```python
from build123d import *

# Parameters (mm, degrees)
SKETCH1_R                     = 39.878
HOUSING_FITTING_EXTRUDE_DEPTH = 17.018
HOUSING_BODY_1_DEPTH          = 19.05
SKETCH3_R                     = 8.509
IMPELLER_BORE_DEPTH           = 17.018
SKETCH4_R                     = 4
SHAFT_BORE_DEPTH              = 70.612
O_RING_CUT_DEPTH              = 1.27
O_RING_CUT_DEPTH_BACK         = 1.27
SKETCH5_R                     = 39.878
SKETCH5_R_2                   = 38.608
SEAL_START                    = 19.05
SKETCH7_R                     = 39.878
SKETCH7_R_2                   = 4
SEAL_SIDE_BODY_EXT_DEPTH      = 19.05
EXT_FILLET_R                  = 5.08
SKETCH10_W                    = 19.05
SKETCH10_H                    = 50.8
DISCHARGE_CUT_DEPTH           = 10.541
SKETCH11_R                    = 19.05
CUT_EXTRUDE1_DEPTH            = 27.94
SKETCH12_R                    = 3.175
CUT_EXTRUDE2_DEPTH            = 19.05
CIRPATTERN1_COUNT             = 8


with BuildPart() as part:
    # Sketch1 → Housing Fitting Extrude (new body)
    with BuildSketch(Plane(origin=(0, 0, 0), x_dir=(0, 0, -1), z_dir=(1, 0, 0))):
        Circle(SKETCH1_R)
    extrude(amount=HOUSING_FITTING_EXTRUDE_DEPTH)

    # Sketch2 → Housing Body 1 (add)
    with BuildSketch(Plane.ZY):
        with BuildLine():
            Line((60.96, 0), (60.96, 60.96))
            Line((60.96, 60.96), (0, 60.96))
            ThreePointArc((0, 60.96), (-43.105229381, 43.105229381), (-60.96, 0))
            Line((-60.96, 0), (-60.96, -54.61))
            Line((-60.96, -54.61), (-60.96, -60.96))
            Line((-60.96, -60.96), (60.96, -60.96))
            Line((60.96, -60.96), (60.96, -54.61))
            Line((60.96, -54.61), (60.96, 0))
        make_face()
    extrude(amount=HOUSING_BODY_1_DEPTH)

    # Sketch3 → Impeller Bore (cut)
    with BuildSketch(Plane(origin=(17.018, 0, 0), x_dir=(0, 0, -1), z_dir=(1, 0, 0))):
        Circle(SKETCH3_R)
    extrude(amount=-IMPELLER_BORE_DEPTH, mode=Mode.SUBTRACT)

    # Sketch4 → Shaft Bore (cut)
    with BuildSketch(Plane(origin=(0, 0, 0), x_dir=(0, 0, -1), z_dir=(1, 0, 0))):
        Circle(SKETCH4_R)
    extrude(amount=-SHAFT_BORE_DEPTH, mode=Mode.SUBTRACT)

    # Sketch5 → O-Ring Cut (cut, two sides: drawn at the far end of the back side and taken through both)
    with BuildSketch(Plane(origin=(8.509, 0, 0), x_dir=(0, 0, -1), z_dir=(1, 0, 0)).offset(-O_RING_CUT_DEPTH_BACK)):
        Circle(SKETCH5_R)
        Circle(SKETCH5_R_2, mode=Mode.SUBTRACT)
    extrude(amount=O_RING_CUT_DEPTH + O_RING_CUT_DEPTH_BACK, mode=Mode.SUBTRACT)

    # Sketch7 → Seal Side Body Ext (add)
    with BuildSketch(Plane.ZY.offset(19.05).offset(SEAL_START)):
        with Locations(Location((0, 0, 0), (0, 0, 180))):
            Circle(SKETCH7_R)
        with Locations(Location((0, 0, 0), (0, 0, 180))):
            Circle(SKETCH7_R_2, mode=Mode.SUBTRACT)
    extrude(amount=-SEAL_SIDE_BODY_EXT_DEPTH)

    # Ext Fillet
    ext_fillet_edges = [part.edges().sort_by_distance(p)[0] for p in [
        (-38.1, 0, 39.878),
        (-19.05, 0, 39.878),
    ]]
    fillet(ext_fillet_edges, radius=EXT_FILLET_R)

    # Sketch10 → Discharge Cut (cut)
    with BuildSketch(Plane.XY.offset(60.96)):
        with Locations((-9.525, 35.56)):
            Rectangle(SKETCH10_W, SKETCH10_H)
    extrude(amount=-DISCHARGE_CUT_DEPTH, mode=Mode.SUBTRACT)

    # Sketch11 → Cut-Extrude1 (cut)
    with BuildSketch(Plane.ZY.offset(38.1)):
        Circle(SKETCH11_R)
    extrude(amount=-CUT_EXTRUDE1_DEPTH, mode=Mode.SUBTRACT)

    # Sketch12 → Cut-Extrude2 (cut)
    with BuildSketch(Plane(origin=(0, 0, 0), x_dir=(0, 0, -1), z_dir=(1, 0, 0))):
        with Locations((-50.419, 0)):
            Circle(SKETCH12_R)
    cut_extrude2 = extrude(amount=-CUT_EXTRUDE2_DEPTH, mode=Mode.SUBTRACT)

    # CirPattern1: Cut-Extrude2 ×8 about axis, 1 skipped
    cirpattern1_axis = Axis((0, 0, 0), (1, 0, 0))
    add([cut_extrude2.rotate(cirpattern1_axis, i * 360 / CIRPATTERN1_COUNT) for i in range(1, CIRPATTERN1_COUNT) if i not in (7,)], mode=Mode.SUBTRACT)


solid = part.part
```
Can you work these out from the model? Positions are in its coordinate system, mm. A direction names the side the tool comes from. Round coordinates to 2 decimals unless told otherwise and drop trailing zeros. Loops run counter-clockwise (first coordinate to the right, second up) from the corner with the lowest first, then second, coordinate; pieces in that order, holes last. Notation, with made-up numbers: (42.5, -11.5) -> (89.5, -11.5) arc R7 ccw to (89.5, -2.5) -> close; hole circle Ø11 at (86, 78.5). An arc over 180 degrees is marked (long way). One line per item, written item: value. Start each with the question number.
1. If we section it at B-B, the plane x = 12: Write out the boundary of the cut face in (y, z).
2. If we section it at A-A, the plane z = -49.5: Write out the boundary of the cut face in (x, y).
3. For pin 1 (1.5 mm diameter, centred on y = 8.5, z = -42, fed in from +X); pin 2 (10 mm diameter, centred on y = 0, z = -50.419, fed in from -X); pin 3 (6 mm diameter, centred on x = -17, y = 43, fed in from +Z), each with a flat end and sliding along its axis, tell me the tip position at first contact or that it passes through.
4. If we section it at C-C, the plane x = -13.5: Give the number of separate pieces and of enclosed holes in the cut face, then the cut area to 3 significant figures.
5. For faces 4 (the flat face through (-10, 36, 50.419)), 5 (the flat face through (-19.05, -40, -28)), 6 (the cylindrical face through (13.348, 33.625, -21.438)), which set-ups out of +Z, -Z, +X, -X, +Y, -Y let a thin tool reach every point of the face, with its end or its side?
6. If I drill on probe 1 along Z at (x, y) = (-14, 2.5); probe 2 along Y at (x, z) = (-24, -7.5); probe 3 along X at (y, z) = (46, 34), over which ranges is the centre line in solid material (lowest first)?
7. If we mould it in two halves opening along Z, with no side actions, what happens to faces 1 (the cylindrical face through (-9.392, -32.624, -36.607)), 2 (the flat face through (-9, -60.96, -1)), 3 (the cylindrical face through (3.569, 33.625, -21.438))? For each: pulls with the +Z half, pulls with the -Z half, needs draft (parallel to the pull), parting line crosses it, or undercut.
Calculated:
1. outline: circle Ø79.76 at (0, 0); hole circle Ø17.02 at (0, 0)
2. outline: (-19.05, -60.96) -> (0, -60.96) -> (0, -3.04) -> (-19.05, -3.04) -> close; (-19.05, 3.04) -> (0, 3.04) -> (0, 35.58) -> (-19.05, 35.58) -> close
3. pin 1: stops at x = 0
3. pin 2: stops at x = -19.05
3. pin 3: stops at z = 50.42
4. separate pieces: 1
4. enclosed holes: 8
4. area: 12,200 mm²
5. face 4: +Z, +X, -X, +Y
5. face 5: -X
5. face 6: +X
6. probe 1: z = -60.91 to -52.38, -48.46 to -18.89, 18.89 to 48.46, 52.38 to 60.96
6. probe 2: y = -39.17 to -17.51, 17.51 to 39.17
6. probe 3: x = -19.05 to 0
7. face 1: undercut
7. face 2: needs draft
7. face 3: parting line crosses it
